Here's how the part is built. I have some questions about the finished solid (model axes, mm). A direction names the side the tool comes from. Give positions to 0.01 mm unless a question says otherwise; leave off trailing zeros. Loops run counter-clockwise (first coordinate to the right, second up) from the corner with the lowest first, then second, coordinate; pieces in that order, holes last. Notation, with made-up numbers: (51.25, 14) - (95.25, 14) arc R26 cw to (95.25, 29) - close; hole circle Ø10 at (-17, 31). An arc over 180 degrees is marked (long way). Use one line per item in the form item = value.
from build123d import *

# Parameters (mm, degrees)
SCHIZZO5_R                   = 1.75
ESTRUSIONE_ESTRUSIONE3_DEPTH = 5
SCHIZZO1_R                   = 1.75
TAGLIO_ESTRUSIONE3_DEPTH     = 2.6
SCHIZZO6_R                   = 1
TAGLIO_ESTRUSIONE4_DEPTH     = 10


with BuildPart() as part:
    # Schizzo5 → Estrusione-Estrusione3 (new body)
    with BuildSketch(Plane.XY):
        with BuildLine():
            Line((-12.11870493, -2.725170944), (10.199561172, -5.744744727))
            ThreePointArc((10.199561172, -5.744744727), (18, -6.270036134), (25.800438828, -5.744744727))
            Line((25.800438828, -5.744744727), (48.11870493, -2.725170944))
            ThreePointArc((48.11870493, -2.725170944), (50.5, 0), (48.11870493, 2.725170944))
            Line((48.11870493, 2.725170944), (25.800438828, 5.744744727))
            ThreePointArc((25.800438828, 5.744744727), (18, 6.270036134), (10.199561172, 5.744744727))
            Line((10.199561172, 5.744744727), (-12.11870493, 2.725170944))
            ThreePointArc((-12.11870493, 2.725170944), (-14.5, 0), (-12.11870493, -2.725170944))
        make_face()
        with Locations((18, 0)):
            Circle(SCHIZZO5_R, mode=Mode.SUBTRACT)
    extrude(amount=ESTRUSIONE_ESTRUSIONE3_DEPTH)

    # Schizzo1 → Taglio-Estrusione3 (cut)
    with BuildSketch(Plane.XY):
        with BuildLine():
            Line((24.948441202, 3.734278154), (34.608428908, 1.712900674))
            ThreePointArc((34.608428908, 1.712900674), (36, 0), (34.608428908, -1.712900674))
            Line((34.608428908, -1.712900674), (24.948441202, -3.734278154))
            ThreePointArc((24.948441202, -3.734278154), (22.862554311, -4.862554311), (21.734278154, -6.948441202))
            Line((21.734278154, -6.948441202), (19.712900674, -16.608428908))
            ThreePointArc((19.712900674, -16.608428908), (18, -18), (16.287099326, -16.608428908))
            Line((16.287099326, -16.608428908), (14.265721846, -6.948441202))
            ThreePointArc((14.265721846, -6.948441202), (13.137445689, -4.862554311), (11.051558798, -3.734278154))
            Line((11.051558798, -3.734278154), (1.391571092, -1.712900674))
            ThreePointArc((1.391571092, -1.712900674), (0, 0), (1.391571092, 1.712900674))
            Line((1.391571092, 1.712900674), (11.051558798, 3.734278154))
            ThreePointArc((11.051558798, 3.734278154), (13.137445689, 4.862554311), (14.265721846, 6.948441202))
            Line((14.265721846, 6.948441202), (16.287099326, 16.608428908))
            ThreePointArc((16.287099326, 16.608428908), (18, 18), (19.712900674, 16.608428908))
            Line((19.712900674, 16.608428908), (21.734278154, 6.948441202))
            ThreePointArc((21.734278154, 6.948441202), (22.862554311, 4.862554311), (24.948441202, 3.734278154))
        make_face()
        with Locations((18, 0)):
            Circle(SCHIZZO1_R, mode=Mode.SUBTRACT)
    extrude(amount=TAGLIO_ESTRUSIONE3_DEPTH, mode=Mode.SUBTRACT)

    # Schizzo6 → Taglio-Estrusione4 (cut)
    with BuildSketch(Plane.XY.offset(5)):
        with Locations((-10.176984684, 0)):
            Circle(SCHIZZO6_R)
        with Locations((46.176984684, 0)):
            Circle(SCHIZZO6_R)
    extrude(amount=-TAGLIO_ESTRUSIONE4_DEPTH, mode=Mode.SUBTRACT)


solid = part.part
(1) For P1, Ø4.5, axis at x = 18, y = 0, coming from the -Z side; P2, Ø3, axis at x = -7, z = 1, coming from the +Y side; P3, Ø3, axis at x = 46.18, y = 0, coming from the -Z side; P4, Ø2, axis at x = 35.5, z = 3.5, coming from the +Y side, each with a flat end and sliding along its axis, tell me the tip position at first contact or that it passes through.
Geometry says:
P1 = 2.6
P2 = 3.62
P3 = 0
P4 = 4.57
(2) For faces 4 (the flat face through (-1.116, -4.214, 2.465)), 5 (the flat face through (18, -3, 2.6)), which set-ups out of +Z, -Z, +X, -X, +Y, -Y let a thin tool reach every point of the face, with its end or its side?
Geometry says:
face_4 = +Z, -Z, -X, -Y
face_5 = -Z
(3) If we section it at A-A (z = 1.7): List the corners of the cut face in (x, y) for me.
Geometry says:
outline = (-12.12, -2.73) - (10.2, -5.74) arc R58.18 ccw to (14, -6.13) arc R4.15 ccw to (11.05, -3.73) - (1.39, -1.71) arc R1.75 cw to (1.39, 1.71) - (11.05, 3.73) arc R4.15 ccw to (14, 6.13) arc R58.18 ccw to (10.2, 5.74) - (-12.12, 2.73) arc R2.75 ccw to start; (22, -6.13) arc R58.18 ccw to (25.8, -5.74) - (48.12, -2.73) arc R2.75 ccw to (48.12, 2.73) - (25.8, 5.74) arc R58.18 ccw to (22, 6.13) arc R4.15 ccw to (24.95, 3.73) - (34.61, 1.71) arc R1.75 cw to (34.61, -1.71) - (24.95, -3.73) arc R4.15 ccw to start; hole circle Ø2 at (-10.18, 0); hole circle Ø2 at (46.18, 0)
(4) If we section it at B-B (y = 0): List the corners of the cut face in (x, z) for me, plus the area to 3 significant figures.
Geometry says:
outline = (-14.5, 0) - (-11.18, 0) - (-11.18, 5) - (-14.5, 5) - close; (-9.18, 0) - (0, 0) - (0, 2.6) - (16.25, 2.6) - (16.25, 5) - (-9.18, 5) - close; (19.75, 2.6) - (36, 2.6) - (36, 0) - (45.18, 0) - (45.18, 5) - (19.75, 5) - close; (47.18, 0) - (50.5, 0) - (50.5, 5) - (47.18, 5) - close
area = 203 mm²
(5) If we section it at C-C (x = 18): List the corners of the cut face in (y, z) for me, plus the area to 3 significant figures.
Geometry says:
outline = (-6.27, 2.6) - (-1.75, 2.6) - (-1.75, 5) - (-6.27, 5) - close; (1.75, 2.6) - (6.27, 2.6) - (6.27, 5) - (1.75, 5) - close
area = 21.7 mm²
(6) If I drill on probe 1 along Z at (x, y) = (32.5, 0.5); probe 2 along Y at (x, z) = (13.5, 2.1); probe 3 along Y at (x, z) = (45.5, 3.15), over which ranges is the centre line in solid material (lowest first)?
Geometry says:
probe_1 = 2.6 to 5
probe_2 = -6.1 to -5.28, 5.28 to 6.1
probe_3 = -3.08 to -0.74, 0.74 to 3.08
(7) If we section it at D-D (x = -1): List the corners of the cut face in (y, z) for me, plus the area to 3 significant figures.
Geometry says:
outline = (-4.23, 0) - (4.23, 0) - (4.23, 5) - (-4.23, 5) - close
area = 42.3 mm²
(8) Thinking about a two-plate mould opening in Y: for faces 1 (the flat face through (37.116, 4.214, 2.465)), 2 (the flat face through (29.85, -2.71, 1.28)), 3 (the flat face through (36.803, -4.256, 2.465)), which applies, pulls with the +Y half, pulls with the -Y half, needs draft (parallel to the pull), parting line crosses it, or undercut?
Geometry says:
face_1 = pulls with the +Y half
face_2 = undercut
face_3 = pulls with the -Y half
